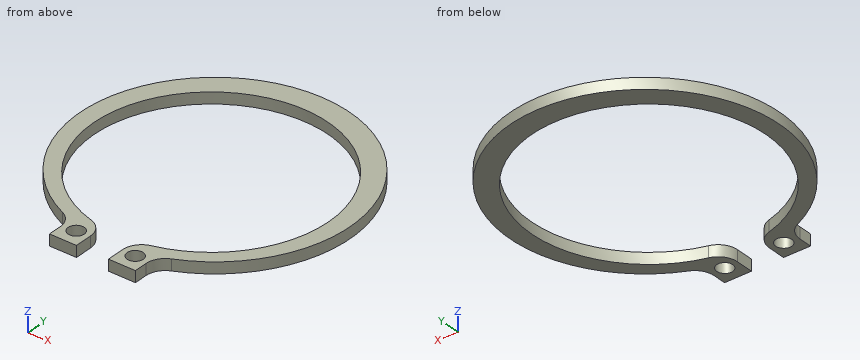
from build123d import *

# Parameters (mm, degrees)
BOSS_EXTRUDE1_DEPTH = 1.75
SKETCH2_R           = 1.25
CUT_EXTRUDE1_DEPTH  = 32.399454524
FILLET1_R           = 3
FILLET2_R           = 3


with BuildPart() as part:
    # Sketch1 → Boss-Extrude1 (new body)
    with BuildSketch(Plane.XY):
        with BuildLine():
            Line((-6.7, -19.152512404), (-6.7, -23.27795619))
            Line((-6.7, -23.27795619), (-2.5, -23.27795619))
            Line((-2.5, -23.27795619), (-2.5, -18.07795619))
            ThreePointArc((-2.5, -18.07795619), (0, 18.25), (2.5, -18.07795619))
            Line((2.5, -18.07795619), (2.5, -23.27795619))
            Line((2.5, -23.27795619), (6.7, -23.27795619))
            Line((6.7, -23.27795619), (6.7, -19.152512404))
            ThreePointArc((6.7, -19.152512404), (0, 21.75), (-6.7, -19.152512404))
        make_face()
    extrude(amount=BOSS_EXTRUDE1_DEPTH)

    # Sketch2 → Cut-Extrude1 (cut, through all)
    with BuildSketch(Plane(origin=(0, 0, 0), x_dir=(-1, 0, 0), z_dir=(0, 0, -1))):
        with Locations((-4.6, -20.67795619)):
            Circle(SKETCH2_R)
    cut_extrude1 = extrude(amount=-CUT_EXTRUDE1_DEPTH, mode=Mode.SUBTRACT)

    # Fillet1
    fillet1_edges = [part.edges().sort_by_distance(p)[0] for p in [
        (6.7, -19.152512404, 0.875),
        (-6.7, -19.152512404, 0.875),
    ]]
    fillet(fillet1_edges, radius=FILLET1_R)

    # Fillet2
    fillet2_edges = [part.edges().sort_by_distance(p)[0] for p in [
        (2.5, -18.07795619, 0.875),
        (-2.5, -18.07795619, 0.875),
    ]]
    fillet(fillet2_edges, radius=FILLET2_R)

    # Mirror1: Cut-Extrude1 across plane
    add(cut_extrude1.mirror(Plane(origin=(0, 0, 0), x_dir=(0, 0, 1), z_dir=(1, 0, 0))), mode=Mode.SUBTRACT)


solid = part.part
Source: CAD feature listing. Evaluate the final solid. Frame: model axes, mm. Coordinates: 2 decimals unless noted, no trailing zeros. Order: outer loops, then holes, each group sorted by start corner. A loop starts at its lowest first (then second) coordinate and runs counter-clockwise, first axis right, second up. Notation, with made-up numbers: M 27,61.25 L 84,61.25 A15 ccw 84,84.25 Z; hole C 51.25,52 d6. An arc over 180 degrees is marked long. Write each question's results on one line, items separated by ' | '. Start each with the question number.
Item 1: Line query: probe 1 along X at (y, z) = (-20, 1.5); probe 2 along Y at (x, z) = (-5, 0.95); probe 3 along Y at (x, z) = (-4.5, 1.05). Output: solid intervals per line, ascending.
Item 2: First-contact query: pin 1 Ø0.9 at (y, z) = (-22, 0.5) entering from -X; pin 2 Ø1 at (x, z) = (6.5, 1) entering from +Y. Flat tips, straight axial feed; report the tip coordinate or a pass-through.
Item 3: Cut plane C-C (z = 0.3). Return loops of the section in (x, y).
Item 4: Cut plane A-A (x = -10). Return loops of the section in (y, z).
Item 5: Cut plane B-B (y = -12.5). Return loops of the section in (x, z).
Item 6: Cut plane D-D (x = 0). Return loops of the section in (y, z).
Checked values:
1) probe 1: x = -6.95 to -5.65, -3.55 to -2.55, 2.55 to 3.55, 5.65 to 6.95 | probe 2: y = -23.28 to -21.86, -19.49 to -17.55, 17.55 to 21.15 | probe 3: y = -23.28 to -21.92, -19.43 to -17.7, 17.69 to 21.26
2) pin 1: stops at x = -6.7 | pin 2: stops at y = 20.87
3) outline: M -8.49,-18.46 A3 cw -6.7,-21.2 L -6.7,-23.28 L -2.5,-23.28 L -2.5,-20.53 A3 ccw -4.72,-17.63 A18.25 cw long 4.72,-17.63 A3 ccw 2.5,-20.53 L 2.5,-23.28 L 6.7,-23.28 L 6.7,-21.2 A3 cw 8.49,-18.46 A21 ccw long Z; hole C -4.6,-20.68 d2.5; hole C 4.6,-20.68 d2.5
4) outline: M -17.72,0 L -15.27,0 L -15.27,1.75 L -17.72,1.75 Z; M 15.27,0 L 19.22,0 L 19.22,1.75 L 15.27,1.75 Z
5) outline: M -16.29,0 L -13.3,0 L -13.3,1.75 L -16.29,1.75 Z; M 13.3,0 L 16.29,0 L 16.29,1.75 L 13.3,1.75 Z
6) outline: M 18.25,0 L 21.75,0 L 21.75,1.75 L 18.25,1.75 Z
